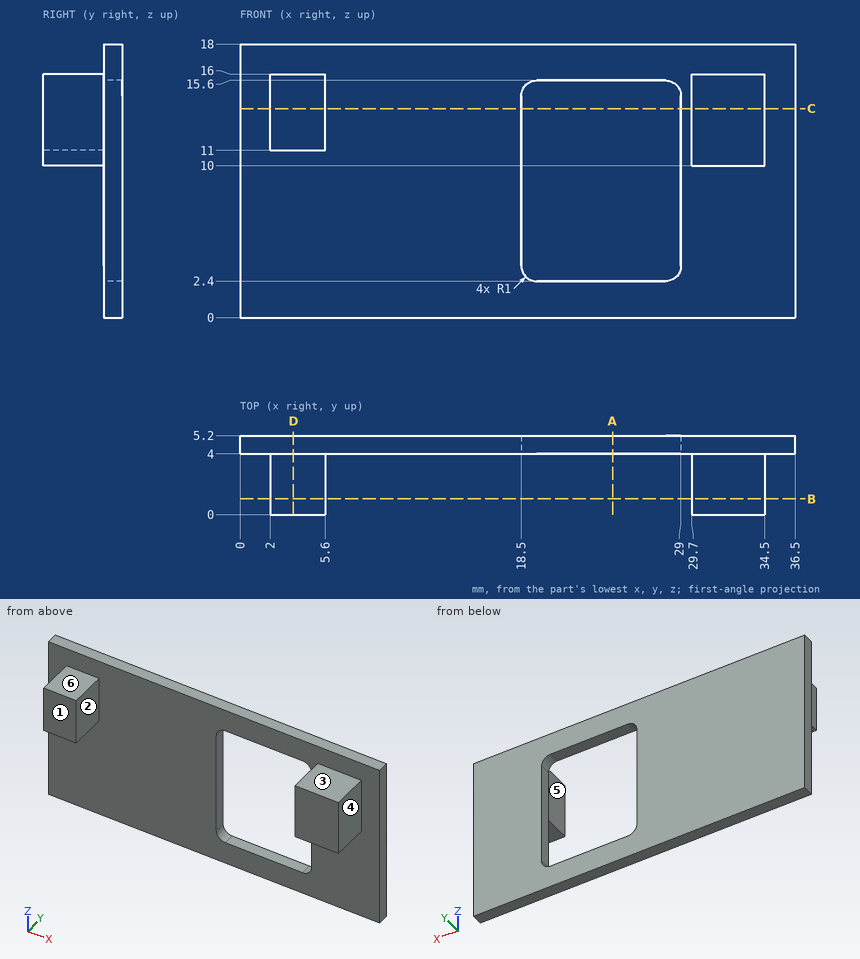
Input: dimensioned drawing with shaded views. Units: mm. Origin: part minimum x, y, z. A direction names the side the tool comes from. Coordinates: 2 decimals unless noted, no trailing zeros. Write each loop counter-clockwise with the first axis right and the second up, starting at its lowest first coordinate (ties: lowest second). Pieces come first, ordered by that corner, then holes. Notation, with made-up numbers: (47.25, 39) -> (65.25, 39) arc R14 cw to (65.25, 54) -> close; hole circle Ø4 at (2.5, -22.5). An arc over 180 degrees is marked (long way). Return JSON: item names as keys, results as strings. Group by question number.
1) Section query A-A, the plane x = 24.5. Return loops of the section in (y, z).
2) Set-up query: the marked faces 1, 2 and 3. Return all of +Z, -Z, +X, -X, +Y, -Y with unobstructed straight access to the full face (end or side cutting, diameter ignored); none if empty.
3) Section query D-D, the plane x = 3.5. Return loops of the section in (y, z).
4) Ray query, line 1 along X through (y, z) = (3.2, 11.25); line 2 along Z through (x, y) = (33.5, 2.55); line 3 along Y through (x, z) = (19, 1.25). Return the intervals inside material, ascending.
5) Section query B-B, the plane y = 1.05. Return loops of the section in (x, z), plus the area to 3 significant figures.
6) Contact query for flat-ended pins moving along their axis: P1, Ø5, axis at x = 23, z = 15, coming from the +Y side; P2, Ø1.8, axis at x = 3, y = 1, coming from the +Z side; P3, Ø2, axis at y = 2.5, z = 13, coming from the +X side; P4, Ø3, axis at x = 3.5, y = 2, coming from the -Z side. Output: stop coordinate, or through.
7) Section query C-C, the plane z = 13.75. Return loops of the section in (x, y), plus the area to 3 significant figures.
8) Mould query, pull axis X, two halves, no side actions, for the marked faces 4, 5 and 6. Classes: +X half, -X half, draft (parallel to the pull), parting line (faces both ways), or undercut.
From the geometry:
{
 "1": {"outline": "(4, 0) -> (5.2, 0) -> (5.2, 2.4) -> (4, 2.4) -> close; (4, 15.6) -> (5.2, 15.6) -> (5.2, 18) -> (4, 18) -> close"},
 "2": {"face 1": "+Z, -Z, +X, -X, -Y", "face 2": "+Z, -Z, -Y", "face 3": "+Z, +X, -X, -Y"},
 "3": {"outline": "(0, 11) -> (4, 11) -> (4, 0) -> (5.2, 0) -> (5.2, 18) -> (4, 18) -> (4, 16) -> (0, 16) -> close"},
 "4": {"line 1": "2 to 5.6, 29.7 to 34.5", "line 2": "10 to 16", "line 3": "4 to 5.2"},
 "5": {"outline": "(2, 11) -> (5.6, 11) -> (5.6, 16) -> (2, 16) -> close; (29.7, 10) -> (34.5, 10) -> (34.5, 16) -> (29.7, 16) -> close", "area": "46.8 mm²"},
 "6": {"P1": "y = 5.2", "P2": "z = 16", "P3": "x = 34.5", "P4": "z = 11"},
 "7": {"outline": "(0, 4) -> (2, 4) -> (2, 0) -> (5.6, 0) -> (5.6, 4) -> (18.5, 4) -> (18.5, 5.2) -> (0, 5.2) -> close; (29, 4) -> (29.7, 4) -> (29.7, 0) -> (34.5, 0) -> (34.5, 4) -> (36.5, 4) -> (36.5, 5.2) -> (29, 5.2) -> close", "area": "64.8 mm²"},
 "8": {"face 4": "+X half", "face 5": "undercut", "face 6": "draft"}
}
